```python
from build123d import *

# Parameters (mm, degrees)
SKETCH1_W           = 76.2
SKETCH1_H           = 25.4
SKETCH1_W_2         = 73.025
SKETCH1_H_2         = 22.225
BOSS_EXTRUDE1_DEPTH = 1803.4
CUT_EXTRUDE1_DEPTH  = 1806.187846181


with BuildPart() as part:
    # Sketch1 → Boss-Extrude1 (new body)
    with BuildSketch(Plane(origin=(0, 0, 0), x_dir=(1, 0, 0), z_dir=(0, 1, 0))):
        with Locations((-38.1, 12.7)):
            Rectangle(SKETCH1_W, SKETCH1_H)
        with Locations((-38.1, 12.7)):
            Rectangle(SKETCH1_W_2, SKETCH1_H_2, mode=Mode.SUBTRACT)
    extrude(amount=BOSS_EXTRUDE1_DEPTH)

    # Sketch2 → Cut-Extrude1 (cut, through all)
    with BuildSketch(Plane.XY):
        with BuildLine():
            Line((-25.4, 1727.2), (-25.4, 1608.697688474))
            ThreePointArc((-25.4, 1608.697688474), (-38.1, 1595.997688474), (-50.8, 1608.697688474))
            Line((-50.8, 1608.697688474), (-50.8, 1727.2))
            ThreePointArc((-50.8, 1727.2), (-38.1, 1739.9), (-25.4, 1727.2))
        make_face()
        with BuildLine():
            Line((-25.4, 1562.1), (-25.4, 1443.597688474))
            ThreePointArc((-25.4, 1443.597688474), (-38.1, 1430.897688474), (-50.8, 1443.597688474))
            Line((-50.8, 1443.597688474), (-50.8, 1562.1))
            ThreePointArc((-50.8, 1562.1), (-38.1, 1574.8), (-25.4, 1562.1))
        make_face()
        with BuildLine():
            Line((-25.4, 1397), (-25.4, 1278.497688474))
            ThreePointArc((-25.4, 1278.497688474), (-38.1, 1265.797688474), (-50.8, 1278.497688474))
            Line((-50.8, 1278.497688474), (-50.8, 1397))
            ThreePointArc((-50.8, 1397), (-38.1, 1409.7), (-25.4, 1397))
        make_face()
        with BuildLine():
            Line((-25.4, 1231.9), (-25.4, 1113.397688474))
            ThreePointArc((-25.4, 1113.397688474), (-38.1, 1100.697688474), (-50.8, 1113.397688474))
            Line((-50.8, 1113.397688474), (-50.8, 1231.9))
            ThreePointArc((-50.8, 1231.9), (-38.1, 1244.6), (-25.4, 1231.9))
        make_face()
        with BuildLine():
            Line((-25.4, 1066.8), (-25.4, 948.297688474))
            ThreePointArc((-25.4, 948.297688474), (-38.1, 935.597688474), (-50.8, 948.297688474))
            Line((-50.8, 948.297688474), (-50.8, 1066.8))
            ThreePointArc((-50.8, 1066.8), (-38.1, 1079.5), (-25.4, 1066.8))
        make_face()
        with BuildLine():
            Line((-25.4, 901.7), (-25.4, 783.197688474))
            ThreePointArc((-25.4, 783.197688474), (-38.1, 770.497688474), (-50.8, 783.197688474))
            Line((-50.8, 783.197688474), (-50.8, 901.7))
            ThreePointArc((-50.8, 901.7), (-38.1, 914.4), (-25.4, 901.7))
        make_face()
        with BuildLine():
            Line((-25.4, 736.6), (-25.4, 618.097688474))
            ThreePointArc((-25.4, 618.097688474), (-38.1, 605.397688474), (-50.8, 618.097688474))
            Line((-50.8, 618.097688474), (-50.8, 736.6))
            ThreePointArc((-50.8, 736.6), (-38.1, 749.3), (-25.4, 736.6))
        make_face()
        with BuildLine():
            Line((-25.4, 571.5), (-25.4, 452.997688474))
            ThreePointArc((-25.4, 452.997688474), (-38.1, 440.297688474), (-50.8, 452.997688474))
            Line((-50.8, 452.997688474), (-50.8, 571.5))
            ThreePointArc((-50.8, 571.5), (-38.1, 584.2), (-25.4, 571.5))
        make_face()
        with BuildLine():
            Line((-25.4, 406.4), (-25.4, 287.897688474))
            ThreePointArc((-25.4, 287.897688474), (-38.1, 275.197688474), (-50.8, 287.897688474))
            Line((-50.8, 287.897688474), (-50.8, 406.4))
            ThreePointArc((-50.8, 406.4), (-38.1, 419.1), (-25.4, 406.4))
        make_face()
        with BuildLine():
            Line((-25.4, 241.3), (-25.4, 122.797688474))
            ThreePointArc((-25.4, 122.797688474), (-38.1, 110.097688474), (-50.8, 122.797688474))
            Line((-50.8, 122.797688474), (-50.8, 241.3))
            ThreePointArc((-50.8, 241.3), (-38.1, 254), (-25.4, 241.3))
        make_face()
    extrude(amount=-CUT_EXTRUDE1_DEPTH, mode=Mode.SUBTRACT)


solid = part.part
```
For this review, take the finished solid that the model builds, in its own axes (mm). Give positions to 0.01 mm unless a question says otherwise; leave off trailing zeros. Write each loop counter-clockwise with the first axis right and the second up, starting at its lowest first coordinate (ties: lowest second). Pieces come first, ordered by that corner, then holes.
Item 1: The part is to be moulded in two halves that separate along X. For faces 1 (the face through (-22, 889, -1.587)), 2 (the face through (-22, 889, -23.812)), 3 (the face through (-56, 889, -25.4)), say which applies: +X half, -X half, draft (parallel to the pull), parting line (faces both ways), or undercut.
Item 2: Wall thickness on probe 1 along Z at (x, y) = (-62, 1134); probe 2 along X at (y, z) = (583, -18.75); probe 3 along X at (y, z) = (1648, -24): over which ranges is each line inside the solid? List them lowest first.
Item 3: Take a section at A-A (y = 194). Give the boundary of the cut face in (x, z).
Item 4: Take a section at C-C (x = -38.1). Give the number of separate pieces and of enclosed holes in the cut face, and give its area (3 significant figures).
Item 5: Take a section at B-B (z = -13.25). Give the boundary of the cut face in (x, y).
Established:
1. face 1: undercut
1. face 2: undercut
1. face 3: draft
2. probe 1: z = -25.4 to -23.81, -1.59 to 0
2. probe 2: x = -76.2 to -74.61, -1.59 to 0
2. probe 3: x = -76.2 to -50.8, -25.4 to 0
3. outline: (-76.2, -25.4) - (-50.8, -25.4) - (-50.8, -23.81) - (-74.61, -23.81) - (-74.61, -1.59) - (-50.8, -1.59) - (-50.8, 0) - (-76.2, 0) - close; (-25.4, -25.4) - (0, -25.4) - (0, 0) - (-25.4, 0) - (-25.4, -1.59) - (-1.59, -1.59) - (-1.59, -23.81) - (-25.4, -23.81) - close
4. separate pieces: 22
4. enclosed holes: 0
4. area: 1,160 mm2
5. outline: (-76.2, 0) - (-74.61, 0) - (-74.61, 1803.4) - (-76.2, 1803.4) - close; (-1.59, 0) - (0, 0) - (0, 1803.4) - (-1.59, 1803.4) - close
